Source: CAD feature listing. Evaluate the final solid. Frame: model axes, mm. Face numbers are marked on the shaded views. A direction names the side the tool comes from. Coordinates: 2 decimals unless noted, no trailing zeros. Order: outer loops, then holes, each group sorted by start corner. A loop starts at its lowest first (then second) coordinate and runs counter-clockwise, first axis right, second up.
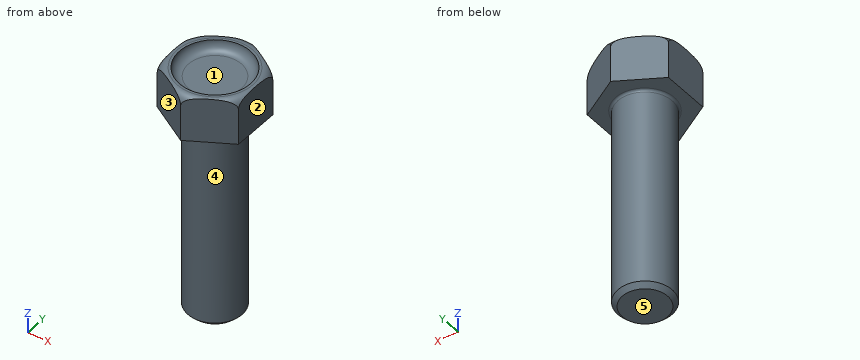
```python
from build123d import *

# Parameters (mm, degrees)
BOSS_EXTRUDE1_DEPTH = 10
SKETCH4_R           = 6
BOSS_EXTRUDE2_DEPTH = 45
CHAMFER1_SIZE       = 1
FILLET1_R           = 0.5
SKETCH6_R           = 7.875
CUT_EXTRUDE1_DEPTH  = 2
FILLET2_R           = 2


with BuildPart() as part:
    # Sketch3 → Boss-Extrude1 (new body)
    with BuildSketch(Plane.XY):
        Polygon((0, 10.392304845), (-9, 5.196152423), (-9, -5.196152423), (0, -10.392304845), (9, -5.196152423), (9, 5.196152423), align=None)
    extrude(amount=BOSS_EXTRUDE1_DEPTH)

    # Sketch4 → Boss-Extrude2 (add)
    with BuildSketch(Plane(origin=(0, 0, 0), x_dir=(-1, 0, 0), z_dir=(0, 0, -1))):
        with Locations(Location((0, 0, 0), (0, 0, 180))):
            Circle(SKETCH4_R)
    extrude(amount=BOSS_EXTRUDE2_DEPTH)

    # Chamfer1
    chamfer1_edges = [part.edges().sort_by_distance(p)[0] for p in [
        (-6, 0, -45),
    ]]
    chamfer(chamfer1_edges, length=CHAMFER1_SIZE)

    # Fillet1
    fillet1_edges = [part.edges().sort_by_distance(p)[0] for p in [
        (-6, 0, 0),
    ]]
    fillet(fillet1_edges, radius=FILLET1_R)

    # Sketch5 → Cut-Revolve1 (revolve, cut)
    with BuildSketch(Plane(origin=(0, 0, 0), x_dir=(0, 0, -1), z_dir=(1, 0, 0))):
        with BuildLine():
            Line((-8, 10.392304845), (-10, 10.392304845))
            Line((-10, 10.392304845), (-10, 8.392304845))
            ThreePointArc((-10, 8.392304845), (-9.414213562, 9.806518408), (-8, 10.392304845))
        make_face()
    revolve(axis=Axis((0, 0, 0), (0, 0, 1)), mode=Mode.SUBTRACT)

    # Sketch6 → Cut-Extrude1 (cut)
    with BuildSketch(Plane.XY.offset(10)):
        Circle(SKETCH6_R)
    extrude(amount=-CUT_EXTRUDE1_DEPTH, mode=Mode.SUBTRACT)

    # Fillet2
    fillet2_edges = [part.edges().sort_by_distance(p)[0] for p in [
        (-7.875, 0, 8),
    ]]
    fillet(fillet2_edges, radius=FILLET2_R - 0.0001)  # a hair under: the kernel refuses the full size


solid = part.part
```
Q1. Pull-direction query (X, two-part tool) for the marked faces 1, 2 and 3; classes: pulls with the +X half, pulls with the -X half, needs draft (parallel to the pull), parting line crosses it, or undercut.
Solutions:
face 1: undercut
face 2: pulls with the +X half
face 3: pulls with the -X half
Q2. Material intervals for line 1 along Z through (x, y) = (3, -1.5); line 2 along Z through (x, y) = (6, -5.75); line 3 along Y through (x, z) = (2, -40), sorted ascending.
Solutions:
line 1: z = -45 to 8
line 2: z = 0 to 10
line 3: y = -5.66 to 5.66
Q3. Pin query (flat end, axial travel): P1, Ø9.5, axis at x = 1.5, y = -1.5, coming from the +Z side; P2, Ø1.5, axis at x = 3.5, z = -11, coming from the +Y side; P3, Ø9.5, axis at x = 0, y = 0, coming from the +Z side. Return the tip coordinate at first contact, or that it passes through.
Solutions:
P1: stops at z = 8.27
P2: stops at y = 5.33
P3: stops at z = 8
Q4. Set-up query: the marked faces 4 and 5. Return all of +Z, -Z, +X, -X, +Y, -Y with unobstructed straight access to the full face (end or side cutting, diameter ignored); none if empty.
Solutions:
face 4: -Z
face 5: -Z, +X, -X, +Y, -Y
Q5. Section query B-B on z = -26. Output: boundary loops of the cut face in (x, y), plus the area to 3 significant figures.
Solutions:
outline: circle Ø12 at (0, 0)
area: 113 mm2
